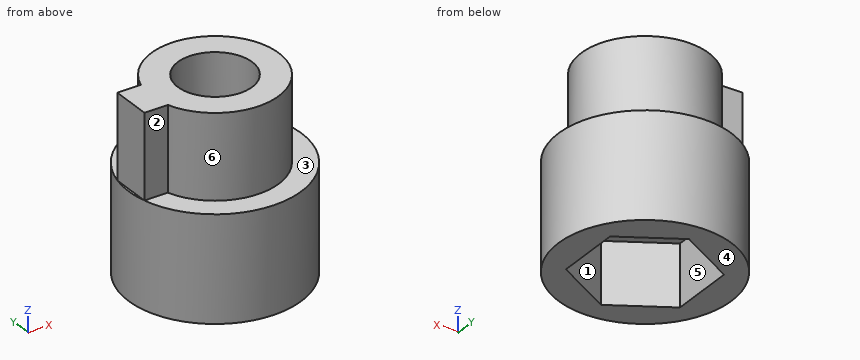
from build123d import *

# Parameters (mm, degrees)
SKETCH1_R           = 4.25
BOSS_EXTRUDE1_DEPTH = 10
SKETCH2_R           = 9.871676656
BOSS_EXTRUDE2_DEPTH = 7
SKETCH3_R           = 9.871676656
SKETCH3_R_2         = 7.3
BOSS_EXTRUDE3_DEPTH = 5
SKETCH4_R           = 4.25
BOSS_EXTRUDE4_DEPTH = 5
CUT_EXTRUDE2_START  = -0.4
CUT_EXTRUDE2_DEPTH  = 0.4


with BuildPart() as part:
    # Sketch1 → Boss-Extrude1 (new body)
    with BuildSketch(Plane.XY):
        with BuildLine():
            Line((-9.6, -2.3), (-6.92820323, -2.3))
            ThreePointArc((-6.92820323, -2.3), (7.3, 0), (-6.92820323, 2.3))
            Line((-6.92820323, 2.3), (-9.6, 2.3))
            Line((-9.6, 2.3), (-9.6, -2.3))
        make_face()
        Circle(SKETCH1_R, mode=Mode.SUBTRACT)
    extrude(amount=BOSS_EXTRUDE1_DEPTH)

    # Sketch2 → Boss-Extrude2 (add)
    with BuildSketch(Plane(origin=(0, 0, 0), x_dir=(-1, 0, 0), z_dir=(0, 0, -1))):
        with Locations(Location((0, 0, 0), (0, 0, 346.526841887))):
            Circle(SKETCH2_R)
        Polygon((0, -7.505553499), (6.5, -3.75277675), (6.5, 3.75277675), (0, 7.505553499), (-6.5, 3.75277675), (-6.5, -3.75277675), align=None, mode=Mode.SUBTRACT)
    extrude(amount=BOSS_EXTRUDE2_DEPTH)

    # Sketch3 → Boss-Extrude3 (add)
    with BuildSketch(Plane.XY):
        with Locations(Location((0, 0, 0), (0, 0, 193.473158113))):
            Circle(SKETCH3_R)
        Circle(SKETCH3_R_2, mode=Mode.SUBTRACT)
    extrude(amount=BOSS_EXTRUDE3_DEPTH)

    # Sketch4 → Boss-Extrude4 (add)
    with BuildSketch(Plane.XY.offset(10)):
        with BuildLine():
            Line((-9.6, -2.3), (-6.92820323, -2.3))
            ThreePointArc((-6.92820323, -2.3), (7.3, 0), (-6.92820323, 2.3))
            Line((-6.92820323, 2.3), (-9.6, 2.3))
            Line((-9.6, 2.3), (-9.6, -2.3))
        make_face()
        Circle(SKETCH4_R, mode=Mode.SUBTRACT)
    extrude(amount=BOSS_EXTRUDE4_DEPTH)

    # Sketch6 → Cut-Extrude2 (cut)
    with BuildSketch(Plane.XY.offset(15).offset(CUT_EXTRUDE2_START)):
        with BuildLine():
            Line((-9.6, 2.3), (-9.6, -2.3))
            Line((-9.6, -2.3), (-6.92820323, -2.3))
            ThreePointArc((-6.92820323, -2.3), (7.3, 0), (-6.92820323, 2.3))
            Line((-6.92820323, 2.3), (-9.6, 2.3))
        make_face()
    extrude(amount=CUT_EXTRUDE2_DEPTH, mode=Mode.SUBTRACT)


solid = part.part
Read the model definition and answer for the solid it produces. Units are mm, in the model's axes. Face numbers are marked on the shaded views. A direction names the side the tool comes from. Give positions to 0.01 mm unless a question says otherwise; leave off trailing zeros. Write each loop counter-clockwise with the first axis right and the second up, starting at its lowest first coordinate (ties: lowest second). Pieces come first, ordered by that corner, then holes. Notation, with made-up numbers: (-5, 0.5) - (53, 0.5) arc R36 cw to (53, 36.5) - close; hole circle Ø11 at (83, -16.5). An arc over 180 degrees is marked (long way). Return JSON: item names as keys, results as strings.
Q1. For a pull along Y with two mould halves and no side action, classify the marked faces 4, 5 and 6 as released by +Y, released by -Y, zero draft, split by the parting line, or undercut.
Reply:
{"face 4": "zero draft", "face 5": "undercut", "face 6": "split by the parting line"}
Q2. For the marked faces 1, 2 and 3, determine the directions among +Z, -Z, +X, -X, +Y, -Y from which every point of the face is accessible in a straight line to the end or side of a thin tool.
Reply:
{"face 1": "-Z", "face 2": "+Z, -X, -Y", "face 3": "+Z"}
Q3. A cutting plane is placed at D-D, the plane z = 12.25. Determine the outline of the cut face in (x, y), and give its area (3 significant figures).
Reply:
{"outline": "(-9.6, -2.3) - (-6.93, -2.3) arc R7.3 ccw (long way) to (-6.93, 2.3) - (-9.6, 2.3) - close; hole circle Ø8.5 at (0, 0)", "area": "122 mm²"}
Q4. A cutting plane is placed at A-A, the plane y = 0. Determine the outline of the cut face in (x, z), and give its area (3 significant figures).
Reply:
{"outline": "(-9.87, -7) - (-6.5, -7) - (-6.5, 0) - (-4.25, 0) - (-4.25, 14.6) - (-9.6, 14.6) - (-9.6, 5) - (-9.87, 5) - close; (4.25, 0) - (6.5, 0) - (6.5, -7) - (9.87, -7) - (9.87, 5) - (7.3, 5) - (7.3, 14.6) - (4.25, 14.6) - close", "area": "184 mm²"}
Q5. A cutting plane is placed at B-B, the plane z = -4.75. Determine the outline of the cut face in (x, y), and give its area (3 significant figures).
Reply:
{"outline": "circle Ø19.74 at (0, 0); hole (-6.5, -3.75) - (0, -7.51) - (6.5, -3.75) - (6.5, 3.75) - (0, 7.51) - (-6.5, 3.75) - close", "area": "160 mm²"}
Q6. Consider line 1 along Y through (x, z) = (-0.25, 11); line 2 along X through (y, z) = (0, 6); line 3 along Y through (x, z) = (0, 3.75). Determine where each line is inside the solid, lowest interval first. Write a range as [from, to].
Reply:
{"line 1": "[-7.3, -4.24], [4.24, 7.3]", "line 2": "[-9.6, -4.25], [4.25, 7.3]", "line 3": "[-9.87, -4.25], [4.25, 9.87]"}
Q7. Given P1, Ø1, axis at x = -7.5, y = 4.5, coming from the +Z side; P2, Ø3, axis at x = -8, z = 8, coming from the -Y side; P3, Ø3, axis at x = -8, z = 10, coming from the +Y side, each flat-ended and moving along its own axis, determine where each tip first touches the part or whether it passes through.
Reply:
{"P1": "z = 5", "P2": "y = -3.32", "P3": "y = 3.32"}
Q8. A cutting plane is placed at C-C, the plane x = -2.25. Determine the outline of the cut face in (y, z), and give its area (3 significant figures).
Reply:
{"outline": "(-9.61, -7) - (-6.21, -7) - (-6.21, 0) - (-3.61, 0) - (-3.61, 14.6) - (-6.94, 14.6) - (-6.94, 5) - (-9.61, 5) - close; (3.61, 0) - (6.21, 0) - (6.21, -7) - (9.61, -7) - (9.61, 5) - (6.94, 5) - (6.94, 14.6) - (3.61, 14.6) - close", "area": "172 mm²"}
